```python
from build123d import *

# Parameters (mm, degrees)
SKETCH1_W           = 20
SKETCH1_H           = 40
BOSS_EXTRUDE1_DEPTH = 5
SKETCH3_W           = 20
SKETCH3_H           = 5
BOSS_EXTRUDE2_DEPTH = 33
SKETCH4_W           = 20
SKETCH4_H           = 3
CUT_EXTRUDE2_DEPTH  = 76.855125074
SKETCH5_W           = 20
SKETCH5_H           = 5
BOSS_EXTRUDE3_DEPTH = 10
SKETCH6_W           = 20
SKETCH6_H           = 5
BOSS_EXTRUDE4_DEPTH = 1.5
SKETCH7_W           = 20
SKETCH7_H           = 5
BOSS_EXTRUDE5_DEPTH = 1.5
SKETCH9_W           = 83
SKETCH9_H           = 5
BOSS_EXTRUDE7_DEPTH = 12.954
SKETCH10_R          = 1
CUT_EXTRUDE3_DEPTH  = 87.978445606
SKETCH11_W          = 32.954
SKETCH11_H          = 1.4986
SKETCH11_H_2        = 1.50368
CUT_EXTRUDE4_DEPTH  = 87.978445606
SKETCH12_R          = 1.575
CUT_EXTRUDE5_DEPTH  = 86.518355536


with BuildPart() as part:
    # Sketch1 → Boss-Extrude1 (new body)
    with BuildSketch(Plane(origin=(0, 0, 0), x_dir=(1, 0, 0), z_dir=(0, 1, 0))):
        with Locations((10, 20)):
            Rectangle(SKETCH1_W, SKETCH1_H)
    extrude(amount=BOSS_EXTRUDE1_DEPTH)

    # Sketch3 → Boss-Extrude2 (add)
    with BuildSketch(Plane(origin=(0, 0, -40), x_dir=(-1, 0, 0), z_dir=(0, 0, -1))):
        with Locations((-10, 2.5)):
            Rectangle(SKETCH3_W, SKETCH3_H)
    extrude(amount=BOSS_EXTRUDE2_DEPTH)

    # Sketch4 → Cut-Extrude2 (cut, through all)
    with BuildSketch(Plane(origin=(0, 5, 0), x_dir=(1, 0, 0), z_dir=(0, 1, 0))):
        with Locations((10, 1.5)):
            Rectangle(SKETCH4_W, SKETCH4_H)
    extrude(amount=-CUT_EXTRUDE2_DEPTH, mode=Mode.SUBTRACT)

    # Sketch5 → Boss-Extrude3 (add)
    with BuildSketch(Plane(origin=(0, 0, -73), x_dir=(-1, 0, 0), z_dir=(0, 0, -1))):
        with Locations((-10, 2.5)):
            Rectangle(SKETCH5_W, SKETCH5_H)
    extrude(amount=BOSS_EXTRUDE3_DEPTH)

    # Sketch6 → Boss-Extrude4 (add)
    with BuildSketch(Plane(origin=(0, 0, -83), x_dir=(-1, 0, 0), z_dir=(0, 0, -1))):
        with Locations((-10, 2.5)):
            Rectangle(SKETCH6_W, SKETCH6_H)
    extrude(amount=BOSS_EXTRUDE4_DEPTH)

    # Sketch7 → Boss-Extrude5 (add)
    with BuildSketch(Plane.XY.offset(-3)):
        with Locations((10, 2.5)):
            Rectangle(SKETCH7_W, SKETCH7_H)
    extrude(amount=BOSS_EXTRUDE5_DEPTH)

    # Sketch9 → Boss-Extrude7 (add)
    with BuildSketch(Plane.ZY):
        with Locations((-43, 2.5)):
            Rectangle(SKETCH9_W, SKETCH9_H)
    extrude(amount=BOSS_EXTRUDE7_DEPTH)

    # Sketch10 → Cut-Extrude3 (cut, through all)
    with BuildSketch(Plane.XZ):
        with Locations(Location((-4.477, -13.5, 0), (0, 0, 270))):
            Circle(SKETCH10_R)
        with Locations(Location((11.523, -13.5, 0), (0, 0, 270))):
            Circle(SKETCH10_R)
        with Locations(Location((11.523, -29.5, 0), (0, 0, 270))):
            Circle(SKETCH10_R)
        with Locations(Location((-4.477, -29.5, 0), (0, 0, 270))):
            Circle(SKETCH10_R)
    extrude(amount=-CUT_EXTRUDE3_DEPTH, mode=Mode.SUBTRACT)

    # Sketch11 → Cut-Extrude4 (cut, through all)
    with BuildSketch(Plane.XZ):
        with Locations((3.523, -2.2493)):
            Rectangle(SKETCH11_W, SKETCH11_H)
        with Locations((3.523, -83.74816)):
            Rectangle(SKETCH11_W, SKETCH11_H_2)
    extrude(amount=-CUT_EXTRUDE4_DEPTH, mode=Mode.SUBTRACT)

    # Sketch12 → Cut-Extrude5 (cut, through all)
    with BuildSketch(Plane.XZ):
        with Locations(Location((-7.954, -7.9986, 0), (0, 0, 270))):
            Circle(SKETCH12_R)
        with Locations(Location((15, -7.9986, 0), (0, 0, 270))):
            Circle(SKETCH12_R)
        with Locations(Location((15, -77.99632, 0), (0, 0, 270))):
            Circle(SKETCH12_R)
        with Locations(Location((-7.954, -77.99632, 0), (0, 0, 270))):
            Circle(SKETCH12_R)
    extrude(amount=-CUT_EXTRUDE5_DEPTH, mode=Mode.SUBTRACT)


solid = part.part
```
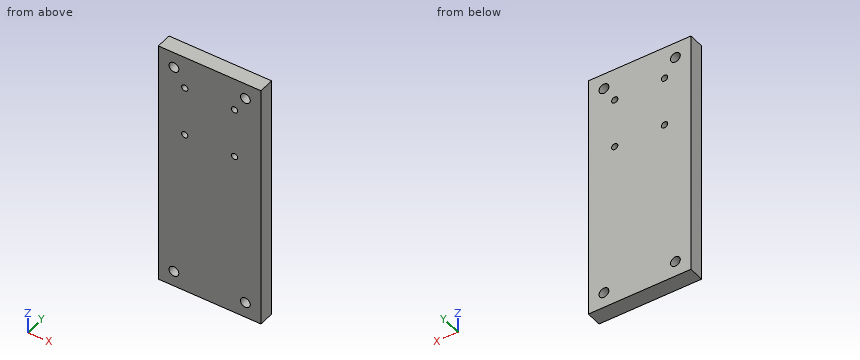
Here's how the part is built. I have some questions about the finished solid (model axes, mm). Round coordinates to 2 decimals unless told otherwise and drop trailing zeros. Write each loop counter-clockwise with the first axis right and the second up, starting at its lowest first coordinate (ties: lowest second). Pieces come first, ordered by that corner, then holes. Notation, with made-up numbers: M -13,3 L 36,3 A16 cw 36,13 Z; hole C 76.5,26 d11. An arc over 180 degrees is marked long. Answer as CSV lines item,"result". Start each with the question number.
1. I need wall thicknesses on probe 1 along X at (y, z) = (1.3, -13.5); probe 2 along Z at (x, y) = (-5, 1.1); probe 3 along Z at (x, y) = (11.5, 0.85). Which ranges of each line are inside material? Lowest first, please.
2. Suppose I cut it at A-A on x = 15. Write out the boundary of the cut face in (y, z).
3. Suppose I cut it at C-C on y = 2.3. Count the separate pieces of the cut face and the enclosed holes in it, then the cut area to 3 significant figures.
4. Suppose I cut it at B-B on z = -29.5. Write out the boundary of the cut face in (x, y).
Check result:
1,probe 1,"x = -12.95 to -5.48, -3.48 to 10.52, 12.52 to 20"
1,probe 2,"z = -83 to -30.35, -28.65 to -14.35, -12.65 to -3"
1,probe 3,"z = -83 to -30.5, -28.5 to -14.5, -12.5 to -3"
2,outline,"M 0,-83 L 5,-83 L 5,-79.57 L 0,-79.57 Z; M 0,-76.42 L 5,-76.42 L 5,-9.57 L 0,-9.57 Z; M 0,-6.42 L 5,-6.42 L 5,-3 L 0,-3 Z"
3,separate pieces,"1"
3,enclosed holes,"8"
3,area,"2,590 mm2"
4,outline,"M -12.95,0 L -5.48,0 L -5.48,5 L -12.95,5 Z; M -3.48,0 L 10.52,0 L 10.52,5 L -3.48,5 Z; M 12.52,0 L 20,0 L 20,5 L 12.52,5 Z"
